Answer from the drawing. Dimensions are ordinates in mm from the lowest x, y and z of the part. A direction names the side the tool comes from. Give positions to 0.01 mm unless a question says otherwise; leave off trailing zeros. Order: outer loops, then holes, each group sorted by start corner. A loop starts at its lowest first (then second) coordinate and runs counter-clockwise, first axis right, second up. Notation, with made-up numbers: (21, -31.5) -> (50, -31.5) arc R14 ccw to (50, -7.5) -> close; hole circle Ø1 at (17, -3.5). An arc over 180 degrees is marked (long way). Answer as CSV lines item,"result". Start each with the question number.
1) Straight lines are drawn through the part: L1, parallel to X at y = 1.3, z = 10; L2, parallel to X at y = 21, z = 12.25; L3, parallel to Z at x = 5.25, y = 2.05. For each, find the intervals that lie inside material, in ascending order. Write a range as from..to.
2) The mould has two halves that part along X. Classify the marked faces 1, 2, 3 and 4: +X half, -X half, draft (parallel to the pull), parting line (faces both ways), or undercut.
3) Find section C-C (y = 7.5). Determine the outline of the cut face in (x, z), and give its area (3 significant figures).
4) Find section D-D (z = 5.75). Determine the outline of the cut face in (x, y).
5) Find section A-A (x = 5.25). Determine the outline of the cut face in (y, z).
6) Find section B-B (z = 10). Determine the outline of the cut face in (x, y).
7) Flat-ended cylindrical pins translate along their axes: pin 1 Ø6 at (y, z) = (19.5, 9) entering from -X; pin 2 Ø11.5 at (x, z) = (40.5, 14.5) entering from +Y; pin 3 Ø11.5 at (x, z) = (3, 6) entering from +Y. Find the tip coordinate at first contact, or state that the pin passes through.
8) For the marked faces 5, 6, 7, 8 and 9, determine the directions among +Z, -Z, +X, -X, +Y, -Y from which every point of the face is accessible in a straight line to the end or side of a thin tool.
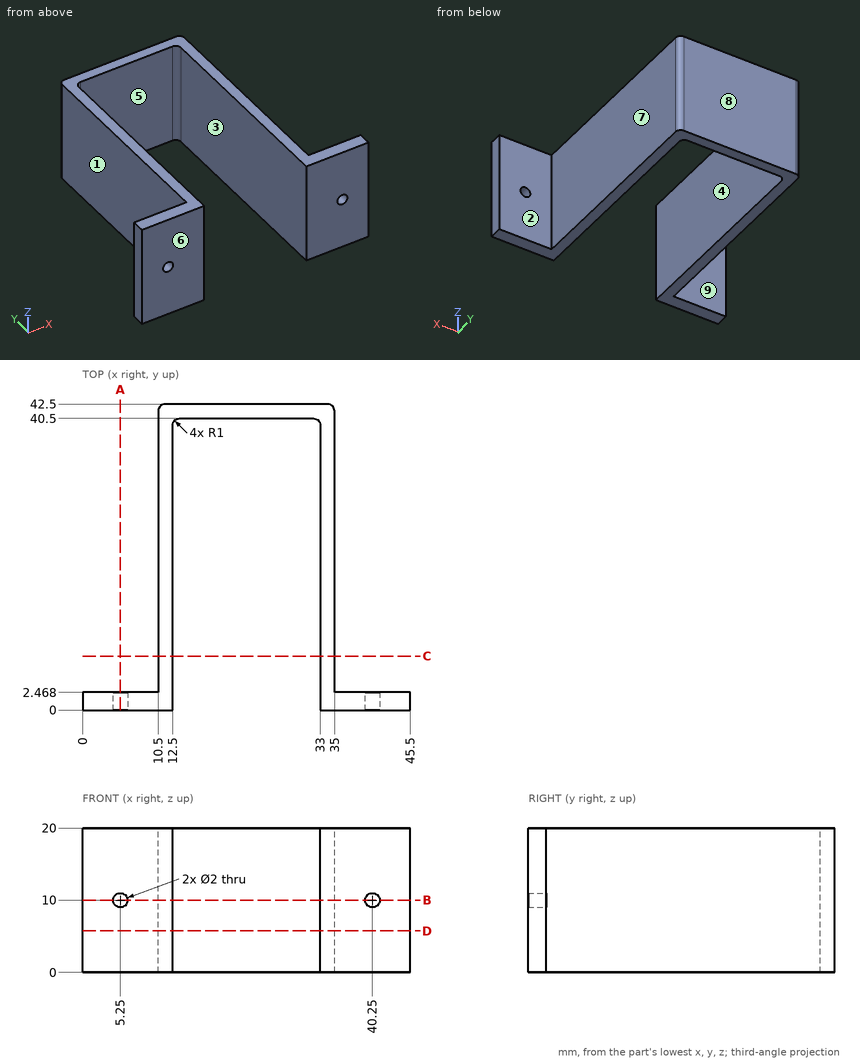
Findings below:
1,L1,"0..4.25, 6.25..12.5, 33..39.25, 41.25..45.5"
1,L2,"10.5..12.5, 33..35"
1,L3,"0..9, 11..20"
2,face 1,"-X half"
2,face 2,"draft"
2,face 3,"undercut"
2,face 4,"undercut"
3,outline,"(10.5, 0) -> (12.5, 0) -> (12.5, 20) -> (10.5, 20) -> close; (33, 0) -> (35, 0) -> (35, 20) -> (33, 20) -> close"
3,area,"80.0 mm²"
4,outline,"(0, 0) -> (12.5, 0) -> (12.5, 39.5) arc R1 cw to (13.5, 40.5) -> (32, 40.5) arc R1 cw to (33, 39.5) -> (33, 0) -> (45.5, 0) -> (45.5, 2.47) -> (35, 2.47) -> (35, 41.5) arc R1 ccw to (34, 42.5) -> (11.5, 42.5) arc R1 ccw to (10.5, 41.5) -> (10.5, 2.47) -> (0, 2.47) -> close"
5,outline,"(0, 0) -> (2.47, 0) -> (2.47, 9) -> (0, 9) -> close; (0, 11) -> (2.47, 11) -> (2.47, 20) -> (0, 20) -> close"
6,outline,"(0, 0) -> (4.25, 0) -> (4.25, 2.47) -> (0, 2.47) -> close; (6.25, 0) -> (12.5, 0) -> (12.5, 39.5) arc R1 cw to (13.5, 40.5) -> (32, 40.5) arc R1 cw to (33, 39.5) -> (33, 0) -> (39.25, 0) -> (39.25, 2.47) -> (35, 2.47) -> (35, 41.5) arc R1 ccw to (34, 42.5) -> (11.5, 42.5) arc R1 ccw to (10.5, 41.5) -> (10.5, 2.47) -> (6.25, 2.47) -> close; (41.25, 0) -> (45.5, 0) -> (45.5, 2.47) -> (41.25, 2.47) -> close"
7,pin 1,"x = 10.5"
7,pin 2,"y = 42.16"
7,pin 3,"y = 2.47"
8,face 5,"+Z, -Z, -Y"
8,face 6,"+Z, -Z, +X, -X, -Y"
8,face 7,"+Z, -Z, +X, +Y"
8,face 8,"+Z, -Z, +X, -X, +Y"
8,face 9,"+Z, -Z, -X, +Y"
